Read the model definition and answer for the solid it produces. Units are mm, in the model's axes. Give positions to 0.01 mm unless a question says otherwise; leave off trailing zeros. Loops run counter-clockwise (first coordinate to the right, second up) from the corner with the lowest first, then second, coordinate; pieces in that order, holes last. Notation, with made-up numbers: (-1, 63) - (31, 63) arc R26 ccw to (31, 94) - close; hole circle Ø7 at (67.25, -16.75). An arc over 180 degrees is marked (long way). Write item = value, one per line.
```python
from build123d import *

# Parameters (mm, degrees)
F0_W     = 11.811
F0_H     = 6.604
F1_DEPTH = 3.175


with BuildPart() as f1:
    # F0 (on Right) → F1 (new body)
    with BuildSketch(Plane.YZ):
        Polygon((60.335764, 22.187536), (33.956723, 45.939331), (5.605423, 45.939331), (5.351423, 45.939331), (4.557673, 45.939331), (4.557673, 49.114331), (-7.348577, 49.114331), (-19.254827, 49.114331), (-19.254827, 45.939331), (-20.048577, 45.939331), (-48.653877, 45.939331), (-48.653877, 3.160534), (-48.653877, -22.239466), (-48.653877, -65.018263), (-14.643277, -65.018263), (-13.849527, -65.018263), (-13.849527, -68.193263), (-1.943277, -68.193263), (9.962973, -68.193263), (9.962973, -65.018263), (10.756723, -65.018263), (11.010723, -65.018263), (44.767323, -65.018263), (65.225091, -49.602229), (65.859237, -49.124843), (67.76977, -51.660206), (77.278524, -44.494846), (86.787278, -37.329486), (84.876745, -34.794122), (85.510433, -34.316128), (85.713286, -34.163267), (105.9682, -18.900094), (79.58916, 4.8517), (78.999288, 5.382823), (81.123778, 7.742308), (72.086951, 15.879103), (63.050124, 24.015898), (60.925635, 21.656414), (60.524522, 22.017577), align=None)
        with Locations((-24.587377, -55.671063)):
            Rectangle(F0_W, F0_H, mode=Mode.SUBTRACT)
    extrude(amount=F1_DEPTH)


solid = f1.part
```
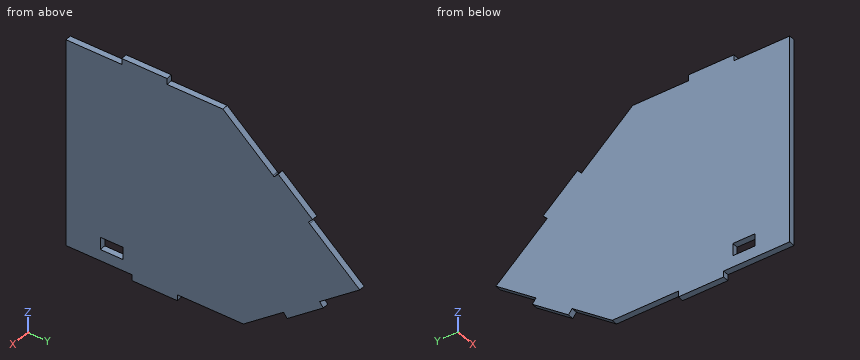
1) A cutting plane is placed at B-B on y = 26. Determine the outline of the cut face in (x, z) (3 decimals), then the cut area to 3 significant figures.
Output:
outline = (0, -65.018) - (3.175, -65.018) - (3.175, 45.939) - (0, 45.939) - close
area = 352 mm²
2) Find the intervals of material crossed by probe 1 along Y at (x, z) = (2.65, -50.5); probe 2 along Z at (x, y) = (1.55, 9); probe 3 along Y at (x, z) = (1.95, 22.5), in increasing order.
Output:
probe_1 = -48.65 to 64.03, 66.9 to 69.31
probe_2 = -68.19 to 45.94
probe_3 = -48.65 to 59.99, 61.69 to 64.73
3) A cutting plane is placed at C-C on z = -13.5. Determine the outline of the cut face in (x, y) (3 decimals).
Output:
outline = (0, -48.654) - (3.175, -48.654) - (3.175, 99.971) - (0, 99.971) - close
4) Each of these flat-tipped pins is pushed along its axis until it touches: P1, Ø1.6, axis at x = 1.5, z = -66.5, coming from the -Y side; P2, Ø1.6, axis at x = 1, y = -23, coming from the +Z side; P3, Ø1, axis at x = 1.5, y = 74.5, coming from the -Z side; P4, Ø1.5, axis at y = 6.5, z = -9, coming from the -X side. Where does it stop, or does it pass through?
Output:
P1 = -13.85
P2 = 45.94
P3 = -46.97
P4 = 0
